from build123d import *

# Parameters (mm, degrees)
F2_R     = 1.524
F3_R     = 3.175
F4_DEPTH = 22.226
F5_COUNT = 6


with BuildPart() as f1:
    # F0 (on Right) → F1 (revolve)
    with BuildSketch(Plane.YZ):
        Polygon((-12.7, 11.1125), (0, 11.1125), (0, 34.1376), (-22.225, 34.1376), (-22.225, 16.6751), (-12.7, 16.6751), align=None)
    revolve(axis=Axis((0, -9.273836258, 0), (0, -1, 0)))

    # F2
    f2_edges = [f1.edges().sort_by_distance(p)[0] for p in [
        (0, -12.7, -16.6751),
    ]]
    fillet(f2_edges, radius=F2_R)

    # F3 (on face) → F4 (cut, through all)
    with BuildSketch(Plane.XZ.offset(22.225)):
        with Locations((0, -26.2001)):
            Circle(F3_R)
    f4 = extrude(amount=-F4_DEPTH, mode=Mode.SUBTRACT)

    # F5: F4 ×6 about axis
    f5_axis = Axis((0, -22.225, 0), (0, -1, 0))
    for i in range(1, F5_COUNT):
        add(f4.rotate(f5_axis, i * 360 / F5_COUNT), mode=Mode.SUBTRACT)


solid = f1.part
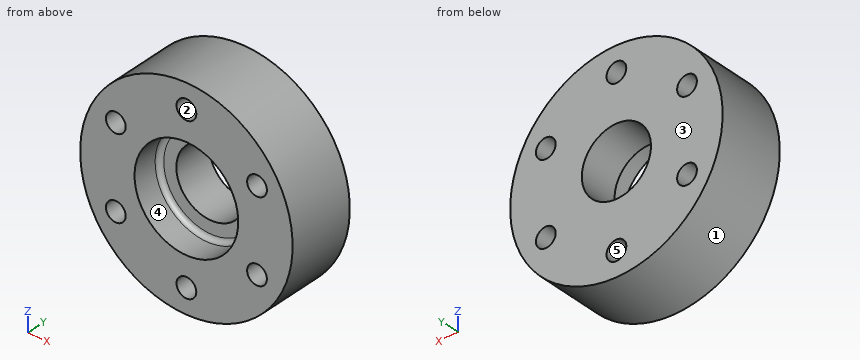
Source: CAD feature listing. Evaluate the final solid. Frame: model axes, mm. Face numbers are marked on the shaded views. A direction names the side the tool comes from. Round coordinates to 2 decimals unless told otherwise and drop trailing zeros. Loops run counter-clockwise (first coordinate to the right, second up) from the corner with the lowest first, then second, coordinate; pieces in that order, holes last. Notation, with made-up numbers: (-26, -9) -> (6, -9) arc R33 cw to (6, 20) -> close; hole circle Ø10 at (20, -5.5). An arc over 180 degrees is marked (long way). Answer as a JSON object with one key per item and string values. Group by question number.
Q1. Section query A-A (z = 0). Output: boundary loops of the cut face in (x, y) (1 decimal), plus the area to 3 significant figures.
Q2. Contact query for flat-ended pins moving along their axis: P1, Ø1.5, axis at y = -13.5, z = -9, coming from the -X side; P2, Ø10, axis at y = -11.5, z = -14.5, coming from the -X side; P3, Ø8, axis at y = -16.5, z = 3, coming from the +X side; P4, Ø5, axis at x = 22.69, z = -13.1, coming from the -Y side. Output: stop coordinate, or through.
Q3. Ray query, line 1 (Z direction, x = 0, y = -14.5); line 2 (Y direction, x = 5, z = 12); line 3 (X direction, y = -17.75, z = 0). Return the intervals inside material, ascending. Write a range as from..to.
Q4. Mould query, pull axis Z, two halves, no side actions, for the marked faces 1, 2 and 3. Classes: pulls with the +Z half, pulls with the -Z half, needs draft (parallel to the pull), parting line crosses it, or undercut.
Q5. Section query D-D (z = -24). Output: boundary loops of the cut face in (x, y) (3 decimals), plus the area to 3 significant figures.
Q6. Section query C-C (y = -4). State how many separate pieces and enclosed holes the cut face has, plus the area to 3 significant figures.
Q7. Access query for the marked faces 4 and 5. Directions: +Z, -Z, +X, -X, +Y, -Y. A direction counts if a zero-diameter tool reaches every point of the face in a straight line with its end or side. Return the directions, or none.
Q8. Section query B-B (x = 0). Output: boundary loops of the cut face in (y, z) (1 decimal).
Completed:
{
 "1": {"outline": "(-34.1, -22.2) -> (-16.7, -22.2) -> (-16.7, -14.2) arc R1.5 cw to (-15.2, -12.7) -> (-11.1, -12.7) -> (-11.1, 0) -> (-34.1, 0) -> close; (11.1, -12.7) -> (15.2, -12.7) arc R1.5 cw to (16.7, -14.2) -> (16.7, -22.2) -> (34.1, -22.2) -> (34.1, 0) -> (11.1, 0) -> close", "area": "918 mm²"},
 "2": {"P1": "x = -33.13", "P2": "x = -32.79", "P3": "x = 34.14", "P4": "through"},
 "3": {"line 1": "-34.14..-29.38, -23.03..-16.68, 16.68..23.03, 29.38..34.14", "line 2": "-12.7..0", "line 3": "-34.14..-16.68, 16.68..34.14"},
 "4": {"face 1": "parting line crosses it", "face 2": "undercut", "face 3": "needs draft"},
 "5": {"outline": "(-24.277, -22.225) -> (-2.289, -22.225) -> (-2.289, 0) -> (-24.277, 0) -> close; (2.289, -22.225) -> (24.277, -22.225) -> (24.277, 0) -> (2.289, 0) -> close", "area": "977 mm²"},
 "6": {"separate pieces": "1", "enclosed holes": "7", "area": "3,080 mm²"},
 "7": {"face 4": "-Y", "face 5": "+Y, -Y"},
 "8": {"outline": "(-22.2, -34.1) -> (0, -34.1) -> (0, -29.4) -> (-22.2, -29.4) -> close; (-22.2, -23) -> (0, -23) -> (0, -11.1) -> (-12.7, -11.1) -> (-12.7, -15.2) arc R1.5 cw to (-14.2, -16.7) -> (-22.2, -16.7) -> close; (-22.2, 16.7) -> (-14.2, 16.7) arc R1.5 cw to (-12.7, 15.2) -> (-12.7, 11.1) -> (0, 11.1) -> (0, 23) -> (-22.2, 23) -> close; (-22.2, 29.4) -> (0, 29.4) -> (0, 34.1) -> (-22.2, 34.1) -> close"}
}
